from build123d import *

# Parameters (mm, degrees)
SKETCH1_R               = 100
BOSS_EXTRUDE1_DEPTH     = 10
BOSS_EXTRUDE2_DEPTH     = 12
CUT_EXTRUDE1_START      = 12
SKETCH2_4_R             = 45
CUT_EXTRUDE1_DEPTH      = 10
CUT_EXTRUDE2_DEPTH      = 142.929559994
CUT_EXTRUDE2_DEPTH_BACK = 142.929559994
SKETCH2_5_R             = 18
SKETCH3_R               = 6
CUT_EXTRUDE3_DEPTH      = 142.929559994
CIRPATTERN1_COUNT       = 6
CIRPATTERN2_COUNT       = 12


with BuildPart() as part:
    # Sketch1 → Boss-Extrude1 (new body)
    with BuildSketch(Plane.XY):
        Circle(SKETCH1_R)
    extrude(amount=BOSS_EXTRUDE1_DEPTH)

    # Sketch2 → Boss-Extrude2 (add)
    with BuildSketch(Plane.XY.offset(10)):
        with BuildLine():
            ThreePointArc((-50.345631284, 62.171676917), (1.396192515, 79.987815613), (52.484722319, 60.376766418))
            ThreePointArc((52.484722319, 60.376766418), (66.748047509, 30.730196137), (55, 0))
            ThreePointArc((55, 0), (50.995112001, -20.603362638), (39.563689019, -38.206210375))
            ThreePointArc((39.563689019, -38.206210375), (29.24031903, -55.29718468), (27.361611466, -75.175409663))
            ThreePointArc((27.361611466, -75.175409663), (0, -80), (-27.361611466, -75.175409663))
            ThreePointArc((-27.361611466, -75.175409663), (-51.676872183, -52.237995658), (-51.683094143, -18.811107883))
            ThreePointArc((-51.683094143, -18.811107883), (-54.947652187, 2.399066305), (-49.846928287, 23.244004396))
            ThreePointArc((-49.846928287, 23.244004396), (-45.650267162, 42.764798591), (-50.345631284, 62.171676917))
        make_face()
    extrude(amount=BOSS_EXTRUDE2_DEPTH)

    # Sketch2<4> → Cut-Extrude1 (cut)
    with BuildSketch(Plane.XY.offset(10).offset(CUT_EXTRUDE1_START)):
        Circle(SKETCH2_4_R)
    extrude(amount=-CUT_EXTRUDE1_DEPTH, mode=Mode.SUBTRACT)

    # Sketch2<5> → Cut-Extrude2 (cut, two sides: drawn at the far end of the back side and taken through both)
    with BuildSketch(Plane.XY.offset(10).offset(-CUT_EXTRUDE2_DEPTH_BACK)):
        Circle(SKETCH2_5_R)
    extrude(amount=CUT_EXTRUDE2_DEPTH + CUT_EXTRUDE2_DEPTH_BACK, mode=Mode.SUBTRACT)

    # Sketch3 → Cut-Extrude3 (cut, through all)
    with BuildSketch(Plane.XY.offset(12)):
        with Locations((32.5, 0)):
            Circle(SKETCH3_R)
    cut_extrude3 = extrude(amount=-CUT_EXTRUDE3_DEPTH, mode=Mode.SUBTRACT)

    # CirPattern1: Cut-Extrude3 ×6 about axis
    cirpattern1_axis = Axis((0, 0, 0), (0, 0, 1))
    for i in range(1, CIRPATTERN1_COUNT):
        add(cut_extrude3.rotate(cirpattern1_axis, i * 360 / CIRPATTERN1_COUNT), mode=Mode.SUBTRACT)

    # Sketch5 → Cut-Revolve2 (revolve, cut)
    with BuildSketch(Plane(origin=(0, 0, 0), x_dir=(1, 0, 0), z_dir=(0, 1, 0))):
        Polygon((83.65, -10), (86.65, -7), (86.65, 0), (90, 0), (90, -10), align=None)
    cut_revolve2 = revolve(axis=Axis((90, 0, 0), (0, 0, 1)), mode=Mode.SUBTRACT)

    # CirPattern2: Cut-Revolve2 ×12 about axis
    cirpattern2_axis = Axis((0, 0, 0), (0, 0, 1))
    for i in range(1, CIRPATTERN2_COUNT):
        add(cut_revolve2.rotate(cirpattern2_axis, i * 360 / CIRPATTERN2_COUNT), mode=Mode.SUBTRACT)


solid = part.part
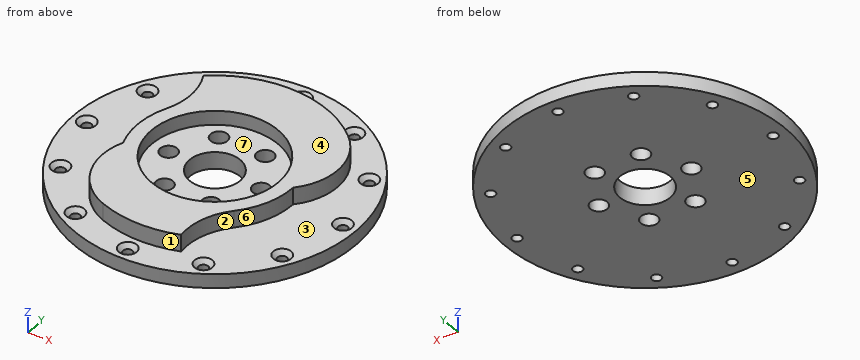
Model file for the job. Use its own axes, mm. Face numbers are marked on the shaded views. A direction names the side the tool comes from. Give positions to 0.01 mm unless a question says otherwise; leave off trailing zeros. Loops run counter-clockwise (first coordinate to the right, second up) from the corner with the lowest first, then second, coordinate; pieces in that order, holes last.
1) Pull direction X, two halves, no side cores. Call the marked faces 5, 6 and 7: +X half, -X half, draft (parallel to the pull), parting line (faces both ways), or undercut.
2) Saw through at A-A (x = -90). Write the cut outline in (y, z).
3) Saw through at C-C (z = 3.75). Count the separate pieces of the cut face and the enclosed holes in it, plus the area to 3 significant figures.
4) Tool access for the marked faces 1, 2, 3 and 4: list every direction of +Z, -Z, +X, -X, +Y, -Y with a clear straight run to the whole face (end or side of a thin tool).
5) Flat gauge pins, fed straight in: pin 1 Ø7.5 at (x, y) = (-77.94, -45) entering from +Z; pin 2 Ø3 at (x, z) = (34.5, 19.5) entering from +Y; pin 3 Ø10 at (x, y) = (-37, -5.5) entering from +Z. Where does each tip first touch, or does it go through?
6) Wall check: line 1 (Z direction, x = -65.5, y = 34.5); line 2 (Y direction, x = -28.5, z = 10.5); line 3 (Y direction, x = 91, z = 2.5). Give the ranges that are in metal, low to high.
7) Saw through at D-D (x = 32.5). Write the cut outline in (y, z).
Answer block:
1. face 5: draft
1. face 6: +X half
1. face 7: undercut
2. outline: (-43.59, 0) - (-3.35, 0) - (-3.35, 7) - (-6.35, 10) - (-43.59, 10) - close; (3.35, 0) - (43.59, 0) - (43.59, 10) - (6.35, 10) - (3.35, 7) - close
3. separate pieces: 1
3. enclosed holes: 19
3. area: 29,300 mm2
4. face 1: +Z, -Y
4. face 2: +Z, +X
4. face 3: +Z
4. face 4: +Z, +X, -X, +Y, -Y
5. pin 1: stops at z = 7.4
5. pin 2: stops at y = 72.88
5. pin 3: stops at z = 12
6. line 1: z = 0 to 10
6. line 2: y = -74.74 to -4.47, 4.47 to 74.75
6. line 3: y = -41.46 to -3.2, 3.2 to 41.46
7. outline: (-94.57, 0) - (-6, 0) - (-6, 12) - (-31.12, 12) - (-31.12, 22) - (-47.8, 22) - (-47.8, 10) - (-94.57, 10) - close; (6, 0) - (94.57, 0) - (94.57, 10) - (73.1, 10) - (73.1, 22) - (31.12, 22) - (31.12, 12) - (6, 12) - close
